Check sheet for the drawn part. Datum: minimum x, y, z corner. Units: mm. Round coordinates to 2 decimals unless told otherwise and drop trailing zeros. Order: outer loops, then holes, each group sorted by start corner. A loop starts at its lowest first (then second) coordinate and runs counter-clockwise, first axis right, second up. Notation, with made-up numbers: (56, 23.5) -> (92, 23.5) arc R12 ccw to (92, 35.5) -> close; hole circle Ø11 at (71, -18.75). An arc over 180 degrees is marked (long way). Answer as CSV lines item,"result". Start each with the question number.
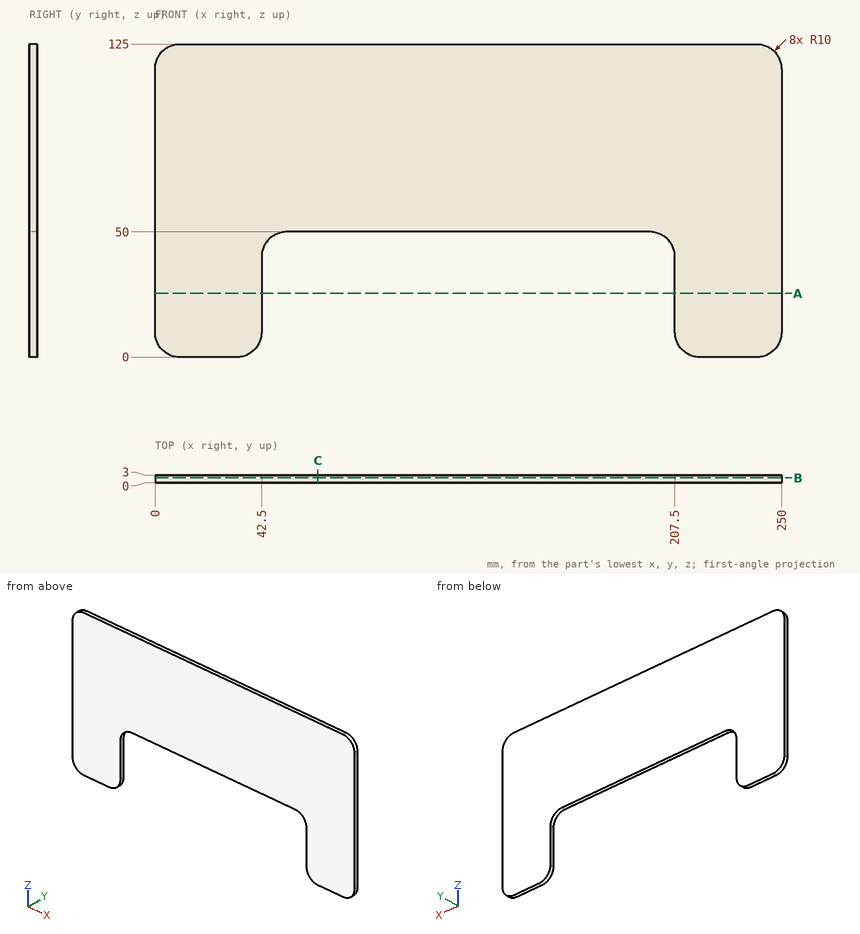
1) Section check A-A on z = 25.5. Record the cut outline in (x, y), then the cut area to 3 significant figures.
2) Material ranges on line 1 along X through (y, z) = (0.4, 22); line 2 along Z through (x, y) = (191.5, 0.95); line 3 along X through (y, z) = (1, 6), recorded low to high.
3) Section check B-B on y = 1.9. Record the cut outline in (x, z), then the cut area to 3 significant figures.
4) Section check C-C on x = 65. Record the cut outline in (y, z), then the cut area to 3 significant figures.
5) Depth check by flat-ended pin: pin 1 Ø0.9 at (x, y) = (95.5, 1.5) entering from -Z. Enter the tip coordinate at first touch or a pass-through.
Solutions:
1,outline,"(0, 0) -> (42.5, 0) -> (42.5, 3) -> (0, 3) -> close; (207.5, 0) -> (250, 0) -> (250, 3) -> (207.5, 3) -> close"
1,area,"255 mm^2"
2,line 1,"x = 0 to 42.5, 207.5 to 250"
2,line 2,"z = 50 to 125"
2,line 3,"x = 0.83 to 41.67, 208.33 to 249.17"
3,outline,"(0, 10) arc R10 ccw to (10, 0) -> (32.5, 0) arc R10 ccw to (42.5, 10) -> (42.5, 40) arc R10 cw to (52.5, 50) -> (197.5, 50) arc R10 cw to (207.5, 40) -> (207.5, 10) arc R10 ccw to (217.5, 0) -> (240, 0) arc R10 ccw to (250, 10) -> (250, 115) arc R10 ccw to (240, 125) -> (10, 125) arc R10 ccw to (0, 115) -> close"
3,area,"22,900 mm^2"
4,outline,"(0, 50) -> (3, 50) -> (3, 125) -> (0, 125) -> close"
4,area,"225 mm^2"
5,pin 1,"stops at z = 50"
